The listing builds one solid part. Answer for the finished solid, in the listing's coordinates (mm). Give positions to 0.01 mm unless a question says otherwise; leave off trailing zeros. Write each loop counter-clockwise with the first axis right and the second up, starting at its lowest first coordinate (ties: lowest second). Pieces come first, ordered by that corner, then holes. Notation, with made-up numbers: (20.25, 22) -> (37.25, 22) arc R13 cw to (37.25, 33) -> close; hole circle Ø6 at (6, -3.5). An arc over 180 degrees is marked (long way). Use CSV: the item, a comma, the result in double quotes. Start each with the question number.
from build123d import *

# Parameters (mm, degrees)
SKETCH1_R           = 7
BOSS_EXTRUDE1_DEPTH = 22
SKETCH2_R           = 4
CUT_EXTRUDE1_DEPTH  = 25.124676164
FILLET1_R           = 1
FILLET2_R           = 1


with BuildPart() as part:
    # Sketch1 → Boss-Extrude1 (new body)
    with BuildSketch(Plane(origin=(0, 0, 0), x_dir=(1, 0, 0), z_dir=(0, 1, 0))):
        with Locations(Location((0, 0, 0), (0, 0, 270))):
            Circle(SKETCH1_R)
    extrude(amount=BOSS_EXTRUDE1_DEPTH)

    # Sketch2 → Cut-Extrude1 (cut, through all)
    with BuildSketch(Plane(origin=(0, 22, 0), x_dir=(1, 0, 0), z_dir=(0, 1, 0))):
        with Locations(Location((0, 0, 0), (0, 0, 270))):
            Circle(SKETCH2_R)
    extrude(amount=-CUT_EXTRUDE1_DEPTH, mode=Mode.SUBTRACT)

    # Fillet1
    fillet1_edges = [part.edges().sort_by_distance(p)[0] for p in [
        (0, 22, -7),
    ]]
    fillet(fillet1_edges, radius=FILLET1_R)

    # Fillet2
    fillet2_edges = [part.edges().sort_by_distance(p)[0] for p in [
        (0, 0, -7),
    ]]
    fillet(fillet2_edges, radius=FILLET2_R)


solid = part.part
Q1. Section B-B on z = 0 is taken. Give the vertices of the cut face in (x, y), then the cut area to 3 significant figures.
Q2. Section A-A on x = 0 is taken. Give the vertices of the cut face in (y, z), then the cut area to 3 significant figures.
Q3. Flat-ended cylindrical pins translate along their axes: pin 1 Ø2 at (x, y) = (-5, 13) entering from -Z; pin 2 Ø1 at (x, y) = (-3, 4) entering from -Z. Find the tip coordinate at first contact, or state that the pin passes through.
Q4. Section C-C on y = 20 is taken. Give the vertices of the cut face in (x, z).
Q5. Straight lines are drawn through the part: L1, parallel to Z at x = 1.75, y = 7.75; L2, parallel to X at y = 12.25, z = 0; L3, parallel to Z at x = 0.25, y = 1.5. For each, find the intervals that lie inside material, in ascending order.
Q6. The mould has two halves that part along X. Classify faces 1 (the face through (-6.834, 10.86, -1.517)), 2 (the face through (-3.92, 0, -1.42)), 3 (the face through (-3.905, 11.154, -0.867)): +X half, -X half, draft (parallel to the pull), parting line (faces both ways), or undercut.
Output:
1,outline,"(-7, 1) arc R1 ccw to (-6, 0) -> (-4, 0) -> (-4, 22) -> (-6, 22) arc R1 ccw to (-7, 21) -> close; (4, 0) -> (6, 0) arc R1 ccw to (7, 1) -> (7, 21) arc R1 ccw to (6, 22) -> (4, 22) -> close"
1,area,"131 mm²"
2,outline,"(0, -6) arc R1 ccw to (1, -7) -> (21, -7) arc R1 ccw to (22, -6) -> (22, -4) -> (0, -4) -> close; (0, 4) -> (22, 4) -> (22, 6) arc R1 ccw to (21, 7) -> (1, 7) arc R1 ccw to (0, 6) -> close"
2,area,"131 mm²"
3,pin 1,"z = -5.74"
3,pin 2,"z = -6.54"
4,outline,"circle Ø14 at (0, 0); hole circle Ø8 at (0, 0)"
5,L1,"-6.78 to -3.6, 3.6 to 6.78"
5,L2,"-7 to -4, 4 to 7"
5,L3,"-7 to -3.99, 3.99 to 7"
6,face 1,"parting line"
6,face 2,"draft"
6,face 3,"undercut"
